Study the drawing (mm; zero at the part's minimum x, y, z) and answer. A direction names the side the tool comes from. Coordinates: 2 decimals unless noted, no trailing zeros. Order: outer loops, then holes, each group sorted by start corner. A loop starts at its lowest first (then second) coordinate and runs counter-clockwise, first axis right, second up.
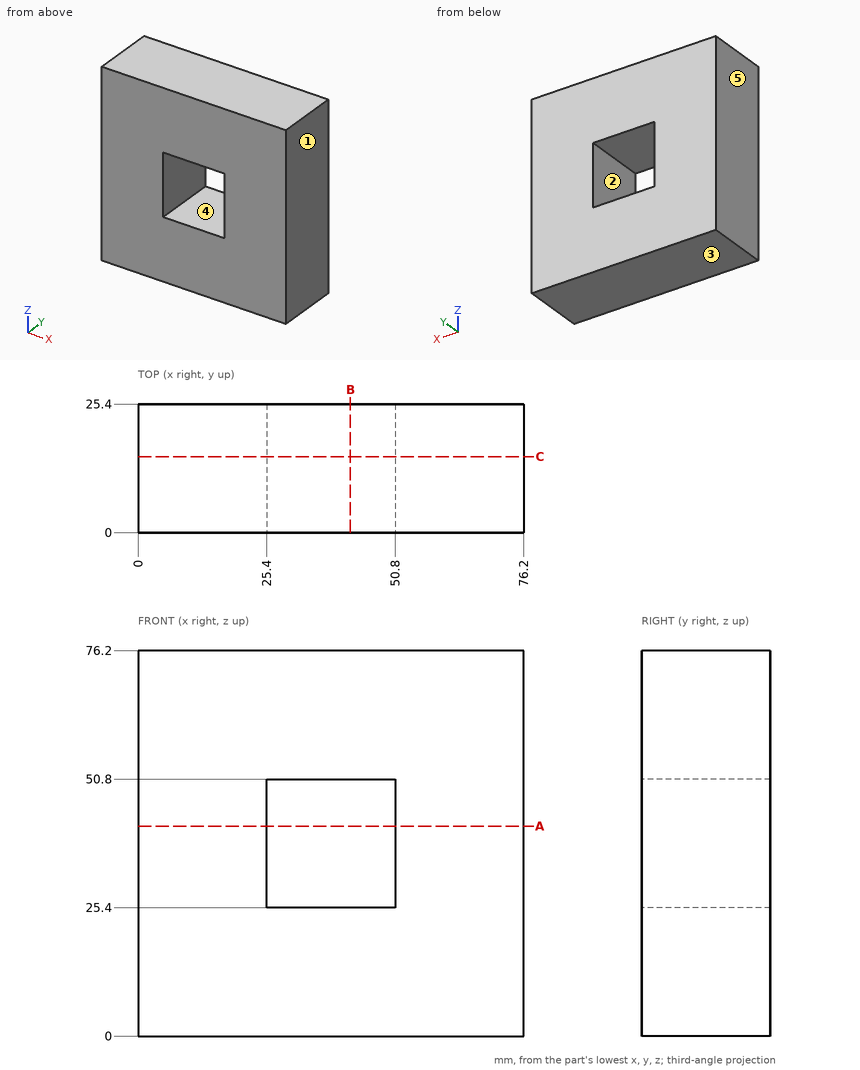
1) A straight line is drawn through the part: line 1 (X direction, y = 2.5, z = 43). Find the intervals that lie inside material, in ascending order.
A:
line 1: x = 0 to 25.4, 50.8 to 76.2
2) A cutting plane is placed at A-A, the plane z = 41.5. Determine the outline of the cut face in (x, y), and give its area (3 significant figures).
A:
outline: (0, 0) - (25.4, 0) - (25.4, 25.4) - (0, 25.4) - close; (50.8, 0) - (76.2, 0) - (76.2, 25.4) - (50.8, 25.4) - close
area: 1,290 mm2
3) Which of the six approach directions +Z, -Z, +X, -X, +Y, -Y give full straight-line access (tool end or side, diameter ignored) to the marked faces 4 and 5?
A:
face 4: +Y, -Y
face 5: +Z, -Z, -X, +Y, -Y
4) Determine the mould class of the marked faces 1, 2 and 3 for opening direction Z: pulls with the +Z half, pulls with the -Z half, needs draft (parallel to the pull), parting line crosses it, or undercut.
A:
face 1: needs draft
face 2: undercut
face 3: pulls with the -Z half
5) A cutting plane is placed at B-B, the plane x = 42. Determine the outline of the cut face in (y, z), and give its area (3 significant figures).
A:
outline: (0, 0) - (25.4, 0) - (25.4, 25.4) - (0, 25.4) - close; (0, 50.8) - (25.4, 50.8) - (25.4, 76.2) - (0, 76.2) - close
area: 1,290 mm2
6) A cutting plane is placed at C-C, the plane y = 15. Determine the outline of the cut face in (x, z).
A:
outline: (0, 0) - (76.2, 0) - (76.2, 76.2) - (0, 76.2) - close; hole (25.4, 25.4) - (50.8, 25.4) - (50.8, 50.8) - (25.4, 50.8) - close
